from build123d import *

# Parameters (mm, degrees)
SKETCH_1_W          = 142
SKETCH_1_H          = 82
EXTRUDE_1_DEPTH     = 15
SHELL_1_T           = -1.5
SKETCH_2_R          = 2.15
CUT_EXTRUDE_1_DEPTH = 15
SKETCH_4_R          = 1.5
CUT_EXTRUDE_2_DEPTH = 15
SKETCH_5_W          = 43
SKETCH_5_H          = 6
CUT_EXTRUDE_3_DEPTH = 15
SKETCH_6_W          = 3
SKETCH_6_H          = 3
EXTRUDE_2_DEPTH     = 2.5
CUT_EXTRUDE_4_REACH = 166.53
SKETCH_7_R          = 0.9
SKETCH_7_R_2        = 0.902391506
FILLET_4_RADIUS     = 1.5
FILLET_4_LENGTH     = 2.5
FILLET_5_RADIUS     = 1.5
FILLET_5_LENGTH     = 2.5
FILLET_6_RADIUS     = 1.5
FILLET_6_LENGTH     = 2.5
FILLET_7_RADIUS     = 1.5
FILLET_7_LENGTH     = 2.5
FILLET_8_R          = 5
FILLET_13_R         = 1.5
SKETCH_8_W          = 139
SKETCH_8_H          = 1
EXTRUDE_7_DEPTH     = 13.5
SKETCH_9_W          = 43
SKETCH_9_H          = 1
EXTRUDE_8_DEPTH     = 7.5
SKETCH_10_W         = 48
SKETCH_10_H         = 1
EXTRUDE_9_DEPTH     = 13.5
FILLET_14_R         = 2


# Some blends are built 0.0001 mm under size
with BuildPart() as part:
    # 草图1 → 凸台-拉伸1 (new body)
    with BuildSketch(Plane(origin=(0, 0, 0), x_dir=(1, 0, 0), z_dir=(0, 1, 0))):
        with Locations((71, -41)):
            Rectangle(SKETCH_1_W, SKETCH_1_H)
    extrude(amount=EXTRUDE_1_DEPTH)

    # 抽壳1
    shell_1_openings = [part.faces().sort_by_distance(p)[0] for p in [
        (71, 15, 41),
    ]]
    offset(amount=SHELL_1_T, openings=shell_1_openings, kind=Kind.INTERSECTION)

    # 草图2 → 切除-拉伸1 (cut)
    with BuildSketch(Plane(origin=(0, 1.5, 0), x_dir=(1, 0, 0), z_dir=(0, 1, 0))):
        with Locations(Location((86.75, -77, 0), (0, 0, 270))):
            Circle(SKETCH_2_R)
        with Locations(Location((55.25, -77, 0), (0, 0, 270))):
            Circle(SKETCH_2_R)
    extrude(amount=-CUT_EXTRUDE_1_DEPTH, mode=Mode.SUBTRACT)

    # 草图4 → 切除-拉伸2 (cut)
    with BuildSketch(Plane(origin=(0, 1.5, 0), x_dir=(1, 0, 0), z_dir=(0, 1, 0))):
        with Locations(Location((5.9, -75.85, 0), (0, 0, 270))):
            Circle(SKETCH_4_R)
        with Locations(Location((136.1, -75.85, 0), (0, 0, 270))):
            Circle(SKETCH_4_R)
        with Locations(Location((5.9, -6.15, 0), (0, 0, 270))):
            Circle(SKETCH_4_R)
        with Locations(Location((136.1, -6.15, 0), (0, 0, 270))):
            Circle(SKETCH_4_R)
    extrude(amount=-CUT_EXTRUDE_2_DEPTH, mode=Mode.SUBTRACT)

    # 草图5 → 切除-拉伸3 (cut)
    with BuildSketch(Plane.XY.offset(82)):
        with Locations((71, 4.5)):
            Rectangle(SKETCH_5_W, SKETCH_5_H)
    extrude(amount=-CUT_EXTRUDE_3_DEPTH, mode=Mode.SUBTRACT)

    # 草图6 → 凸台-拉伸2 (add)
    with BuildSketch(Plane(origin=(0, 11, 0), x_dir=(1, 0, 0), z_dir=(0, 1, 0))):
        with Locations((3, -69)):
            Rectangle(SKETCH_6_W, SKETCH_6_H)
        with Locations((3, -13)):
            Rectangle(SKETCH_6_W, SKETCH_6_H)
        with Locations((139, -13)):
            Rectangle(SKETCH_6_W, SKETCH_6_H)
        with Locations((139, -69)):
            Rectangle(SKETCH_6_W, SKETCH_6_H)
    extrude(amount=EXTRUDE_2_DEPTH)

    # 草图7 → 切除-拉伸4 (cut, up to next)
    with BuildSketch(Plane(origin=(0, 13.5, 0), x_dir=(1, 0, 0), z_dir=(0, 1, 0)), mode=Mode.PRIVATE) as cut_extrude_4_sk1:
        with Locations(Location((3, -13, 0), (0, 0, 270))):
            Circle(SKETCH_7_R)
    cut_extrude_4_tool1 = extrude(cut_extrude_4_sk1.sketch, amount=-CUT_EXTRUDE_4_REACH, mode=Mode.PRIVATE) & part.part
    # 草图7 → 切除-拉伸4 (cut, up to next)
    with BuildSketch(Plane(origin=(0, 13.5, 0), x_dir=(1, 0, 0), z_dir=(0, 1, 0)), mode=Mode.PRIVATE) as cut_extrude_4_sk2:
        with Locations(Location((3, -69, 0), (0, 0, 270))):
            Circle(SKETCH_7_R_2)
    cut_extrude_4_tool2 = extrude(cut_extrude_4_sk2.sketch, amount=-CUT_EXTRUDE_4_REACH, mode=Mode.PRIVATE) & part.part
    # 草图7 → 切除-拉伸4 (cut, up to next)
    with BuildSketch(Plane(origin=(0, 13.5, 0), x_dir=(1, 0, 0), z_dir=(0, 1, 0)), mode=Mode.PRIVATE) as cut_extrude_4_sk3:
        with Locations(Location((139, -69, 0), (0, 0, 270))):
            Circle(SKETCH_7_R)
    cut_extrude_4_tool3 = extrude(cut_extrude_4_sk3.sketch, amount=-CUT_EXTRUDE_4_REACH, mode=Mode.PRIVATE) & part.part
    # 草图7 → 切除-拉伸4 (cut, up to next)
    with BuildSketch(Plane(origin=(0, 13.5, 0), x_dir=(1, 0, 0), z_dir=(0, 1, 0)), mode=Mode.PRIVATE) as cut_extrude_4_sk4:
        with Locations(Location((139, -13, 0), (0, 0, 270))):
            Circle(SKETCH_7_R)
    cut_extrude_4_tool4 = extrude(cut_extrude_4_sk4.sketch, amount=-CUT_EXTRUDE_4_REACH, mode=Mode.PRIVATE) & part.part
    add(cut_extrude_4_tool1.solids().sort_by_distance((3, 13.5, 13))[0], mode=Mode.SUBTRACT)
    add(cut_extrude_4_tool2.solids().sort_by_distance((3, 13.5, 69))[0], mode=Mode.SUBTRACT)
    add(cut_extrude_4_tool3.solids().sort_by_distance((139, 13.5, 69))[0], mode=Mode.SUBTRACT)
    add(cut_extrude_4_tool4.solids().sort_by_distance((139, 13.5, 13))[0], mode=Mode.SUBTRACT)

    # 圆角4: full round fillet: the end face becomes a half cylinder, R = half its width
    fillet_4_face = Plane((4.5, 12.25, 13), x_dir=(0, -1, 0), z_dir=(1, 0, 0))  # on the end face: x along it, z out of the body
    fillet_4_slab = fillet_4_face.offset(-FILLET_4_RADIUS / 2) * Box(FILLET_4_LENGTH, 2 * FILLET_4_RADIUS, FILLET_4_RADIUS, mode=Mode.PRIVATE)  # the body's end, R deep
    fillet_4_round = Plane((3, 12.25, 13), x_dir=(1, 0, 0), z_dir=(0, -1, 0)) * Cylinder(FILLET_4_RADIUS, FILLET_4_LENGTH, mode=Mode.PRIVATE)  # its axis R under the face
    add(fillet_4_slab - fillet_4_round, mode=Mode.SUBTRACT)

    # 圆角5: full round fillet: the end face becomes a half cylinder, R = half its width
    fillet_5_face = Plane((4.5, 12.25, 69), x_dir=(0, -1, 0), z_dir=(1, 0, 0))  # on the end face: x along it, z out of the body
    fillet_5_slab = fillet_5_face.offset(-FILLET_5_RADIUS / 2) * Box(FILLET_5_LENGTH, 2 * FILLET_5_RADIUS, FILLET_5_RADIUS, mode=Mode.PRIVATE)  # the body's end, R deep
    fillet_5_round = Plane((3, 12.25, 69), x_dir=(1, 0, 0), z_dir=(0, -1, 0)) * Cylinder(FILLET_5_RADIUS, FILLET_5_LENGTH, mode=Mode.PRIVATE)  # its axis R under the face
    add(fillet_5_slab - fillet_5_round, mode=Mode.SUBTRACT)

    # 圆角6: full round fillet: the end face becomes a half cylinder, R = half its width
    fillet_6_face = Plane((137.5, 12.25, 13), x_dir=(0, -1, 0), z_dir=(-1, 0, 0))  # on the end face: x along it, z out of the body
    fillet_6_slab = fillet_6_face.offset(-FILLET_6_RADIUS / 2) * Box(FILLET_6_LENGTH, 2 * FILLET_6_RADIUS, FILLET_6_RADIUS, mode=Mode.PRIVATE)  # the body's end, R deep
    fillet_6_round = Plane((139, 12.25, 13), x_dir=(-1, 0, 0), z_dir=(0, -1, 0)) * Cylinder(FILLET_6_RADIUS, FILLET_6_LENGTH, mode=Mode.PRIVATE)  # its axis R under the face
    add(fillet_6_slab - fillet_6_round, mode=Mode.SUBTRACT)

    # 圆角7: full round fillet: the end face becomes a half cylinder, R = half its width
    fillet_7_face = Plane((137.5, 12.25, 69), x_dir=(0, -1, 0), z_dir=(-1, 0, 0))  # on the end face: x along it, z out of the body
    fillet_7_slab = fillet_7_face.offset(-FILLET_7_RADIUS / 2) * Box(FILLET_7_LENGTH, 2 * FILLET_7_RADIUS, FILLET_7_RADIUS, mode=Mode.PRIVATE)  # the body's end, R deep
    fillet_7_round = Plane((139, 12.25, 69), x_dir=(-1, 0, 0), z_dir=(0, -1, 0)) * Cylinder(FILLET_7_RADIUS, FILLET_7_LENGTH, mode=Mode.PRIVATE)  # its axis R under the face
    add(fillet_7_slab - fillet_7_round, mode=Mode.SUBTRACT)

    # 圆角8
    fillet_8_edges = [part.edges().sort_by_distance(p)[0] for p in [
        (0, 7.5, 0),
        (142, 7.5, 0),
        (142, 7.5, 82),
        (0, 7.5, 82),
    ]]
    fillet(fillet_8_edges, radius=FILLET_8_R)

    # 圆角13
    fillet_13_edges = [part.edges().sort_by_distance(p)[0] for p in [
        (71, 0, 82),
        (0, 0, 41),
        (71, 0, 0),
        (142, 0, 41),
        (140.535533906, 0, 80.535533906),
        (140.535533906, 0, 1.464466094),
        (1.464466094, 0, 1.464466094),
        (1.464466094, 0, 80.535533906),
    ]]
    fillet(fillet_13_edges, radius=FILLET_13_R - 0.0001)  # a hair under: the kernel refuses the full size

    # 草图8 → 凸台-拉伸7 (add)
    with BuildSketch(Plane(origin=(0, 15, 0), x_dir=(1, 0, 0), z_dir=(0, 1, 0))):
        with Locations((71, -2)):
            Rectangle(SKETCH_8_W, SKETCH_8_H)
    extrude(amount=-EXTRUDE_7_DEPTH)

    # 草图9 → 凸台-拉伸8 (add)
    with BuildSketch(Plane(origin=(0, 15, 0), x_dir=(1, 0, 0), z_dir=(0, 1, 0))):
        with Locations((71, -80)):
            Rectangle(SKETCH_9_W, SKETCH_9_H)
    extrude(amount=-EXTRUDE_8_DEPTH)

    # 草图10 → 凸台-拉伸9 (add)
    with BuildSketch(Plane(origin=(0, 15, 0), x_dir=(1, 0, 0), z_dir=(0, 1, 0))):
        with Locations((25.5, -80)):
            Rectangle(SKETCH_10_W, SKETCH_10_H)
        with Locations((116.5, -80)):
            Rectangle(SKETCH_10_W, SKETCH_10_H)
    extrude(amount=-EXTRUDE_9_DEPTH)

    # 圆角14
    # the kernel refuses this fillet: 2 mm, written as the material it takes off along each edge
    with BuildSketch(Plane(origin=(5, 15, 77), x_dir=(0, 0, 1), z_dir=(1, 0, 0))) as fillet_14_piece_1:
        with BuildLine():
            CenterArc((5 - FILLET_14_R, FILLET_14_R), FILLET_14_R, 270, 90)
            Line((5 - FILLET_14_R, 0), (5, 0))
            Line((5, 0), (5, FILLET_14_R))
        make_face()
    revolve(axis=Axis((5, 15, 77), (0, -1, 0)), revolution_arc=90, mode=Mode.SUBTRACT)
    with BuildSketch(Plane(origin=(5, 15, 5), x_dir=(0, 0, -1), z_dir=(1, 0, 0))) as fillet_14_piece_2:
        with BuildLine():
            CenterArc((5 - FILLET_14_R, -FILLET_14_R), FILLET_14_R, 0, 90)
            Line((5, -FILLET_14_R), (5, 0))
            Line((5, 0), (5 - FILLET_14_R, 0))
        make_face()
    revolve(axis=Axis((5, 15, 5), (0, 1, 0)), revolution_arc=90, mode=Mode.SUBTRACT)
    with BuildSketch(Plane(origin=(5, 15, 0), x_dir=(0, -1, 0), z_dir=(1, 0, 0)), Plane(origin=(137, 15, 82), x_dir=(0, -1, 0), z_dir=(-1, 0, 0))) as fillet_14_piece_3:
        with BuildLine():
            CenterArc((FILLET_14_R, -FILLET_14_R), FILLET_14_R, 90, 90)
            Line((0, -FILLET_14_R), (0, 0))
            Line((0, 0), (FILLET_14_R, 0))
        make_face()
    extrude(amount=132, mode=Mode.SUBTRACT)
    with BuildSketch(Plane(origin=(137, 15, 5), x_dir=(0, 0, -1), z_dir=(-1, 0, 0))) as fillet_14_piece_4:
        with BuildLine():
            CenterArc((5 - FILLET_14_R, FILLET_14_R), FILLET_14_R, 270, 90)
            Line((5 - FILLET_14_R, 0), (5, 0))
            Line((5, 0), (5, FILLET_14_R))
        make_face()
    revolve(axis=Axis((137, 15, 5), (0, -1, 0)), revolution_arc=90, mode=Mode.SUBTRACT)
    with BuildSketch(Plane(origin=(137, 15, 77), x_dir=(0, 0, 1), z_dir=(-1, 0, 0))) as fillet_14_piece_5:
        with BuildLine():
            CenterArc((5 - FILLET_14_R, -FILLET_14_R), FILLET_14_R, 0, 90)
            Line((5 - FILLET_14_R, 0), (5, 0))
            Line((5, 0), (5, -FILLET_14_R))
        make_face()
    revolve(axis=Axis((137, 15, 77), (0, 1, 0)), revolution_arc=90, mode=Mode.SUBTRACT)
    with BuildSketch(Plane(origin=(142, 15, 5), x_dir=(0, -1, 0), z_dir=(0, 0, 1)), Plane(origin=(0, 15, 77), x_dir=(0, -1, 0), z_dir=(0, 0, -1))) as fillet_14_piece_6:
        with BuildLine():
            CenterArc((FILLET_14_R, -FILLET_14_R), FILLET_14_R, 90, 90)
            Line((0, -FILLET_14_R), (0, 0))
            Line((0, 0), (FILLET_14_R, 0))
        make_face()
    extrude(amount=72, mode=Mode.SUBTRACT)


solid = part.part
Can you work these out from the model? Positions are in its coordinate system, mm. A direction names the side the tool comes from. Give positions to 0.01 mm unless a question says otherwise; leave off trailing zeros. Loops run counter-clockwise (first coordinate to the right, second up) from the corner with the lowest first, then second, coordinate; pieces in that order, holes last. Notation, with made-up numbers: (58.5, 68) - (112.5, 68) arc R29 cw to (112.5, 96) - close; hole circle Ø1 at (-37, -5). An arc over 180 degrees is marked (long way). One line per item, written item: value.
(1) If we section it at B-B, the plane y = 5.25: List the corners of the cut face in (x, z) for me, plus the area to 3 significant figures.
Verdict:
outline: (0, 5) arc R5 ccw to (5, 0) - (137, 0) arc R5 ccw to (142, 5) - (142, 77) arc R5 ccw to (137, 82) - (92.5, 82) - (92.5, 79.5) - (140.5, 79.5) - (140.5, 2.5) - (1.5, 2.5) - (1.5, 79.5) - (49.5, 79.5) - (49.5, 82) - (5, 82) arc R5 ccw to (0, 77) - close
area: 812 mm^2
(2) If we section it at C-C, the plane z = 25.5: List the corners of the cut face in (x, y) for me, plus the area to 3 significant figures.
Verdict:
outline: (0, 1.5) arc R1.5 ccw to (1.5, 0) - (140.5, 0) arc R1.5 ccw to (142, 1.5) - (142, 13) arc R2 ccw to (140.5, 14.94) - (140.5, 1.5) - (1.5, 1.5) - (1.5, 14.94) arc R2 ccw to (0, 13) - close
area: 251 mm^2
(3) If we mould it in two halves opening along Z, with no side actions, what happens to faces 5 (the face through (2, 11, 70)), 6 (the face through (1, 7, 2)), 7 (the face through (1, 7, 80)), 8 (the face through (140, 13.5, 14))? For each: released by +Z, released by -Z, zero draft, split by the parting line, or undercut.
Verdict:
face 5: undercut
face 6: released by -Z
face 7: released by +Z
face 8: undercut
(4) I'm going to push flat-ended pins straight in: pin 1 (1.2 mm diameter, centred on x = 2, y = 13, fed in from -Z); pin 2 (2.5 mm diameter, centred on x = 136.1, z = 6.15, fed in from +Y); pin 3 (0.9 mm diameter, centred on x = 2.5, z = 13, fed in from +Y); pin 4 (1.6 mm diameter, centred on x = 139.5, y = 12.5, fed in from -Z). Where does each tip first touch, or does it pass through?
Verdict:
pin 1: z = 0.61
pin 2: through
pin 3: y = 13.5
pin 4: z = 0.3
(5) On a 3-axis mill with a long thin cutter (end or side, diameter ignored), from which of +Z, -Z, +X, -X, +Y, -Y can I reach the whole of each face in a straight line? I mean faces 1 (the face through (0, 7, 42)), 2 (the face through (70, 8, 79.5)), 3 (the face through (2, 11, 14)), 4 (the face through (92.5, 4, 81)). Say none if no direction works.
Verdict:
face 1: +Z, -Z, -X, +Y, -Y
face 2: +Y
face 3: none
face 4: +Z
(6) I need wall thicknesses on line 1 along X through (y, z) = (12.5, 69); line 2 along X through (y, z) = (13.25, 65); line 3 along Z through (x, y) = (115, 11). Which ranges of each line are inside material? Lowest first, please.
Verdict:
line 1: 0 to 2.1, 3.9 to 4.5, 137.5 to 138.1, 139.9 to 142
line 2: 0.02 to 1.5, 140.5 to 141.98
line 3: 0 to 2.5, 79.5 to 82
(7) If we section it at D-D, the plane x = 33: List the corners of the cut face in (y, z) for me.
Verdict:
outline: (0, 1.5) arc R1.5 ccw to (1.5, 0) - (13, 0) arc R2 ccw to (15, 2) - (15, 2.5) - (1.5, 2.5) - (1.5, 79.5) - (15, 79.5) - (15, 80) arc R2 ccw to (13, 82) - (1.5, 82) arc R1.5 ccw to (0, 80.5) - close
